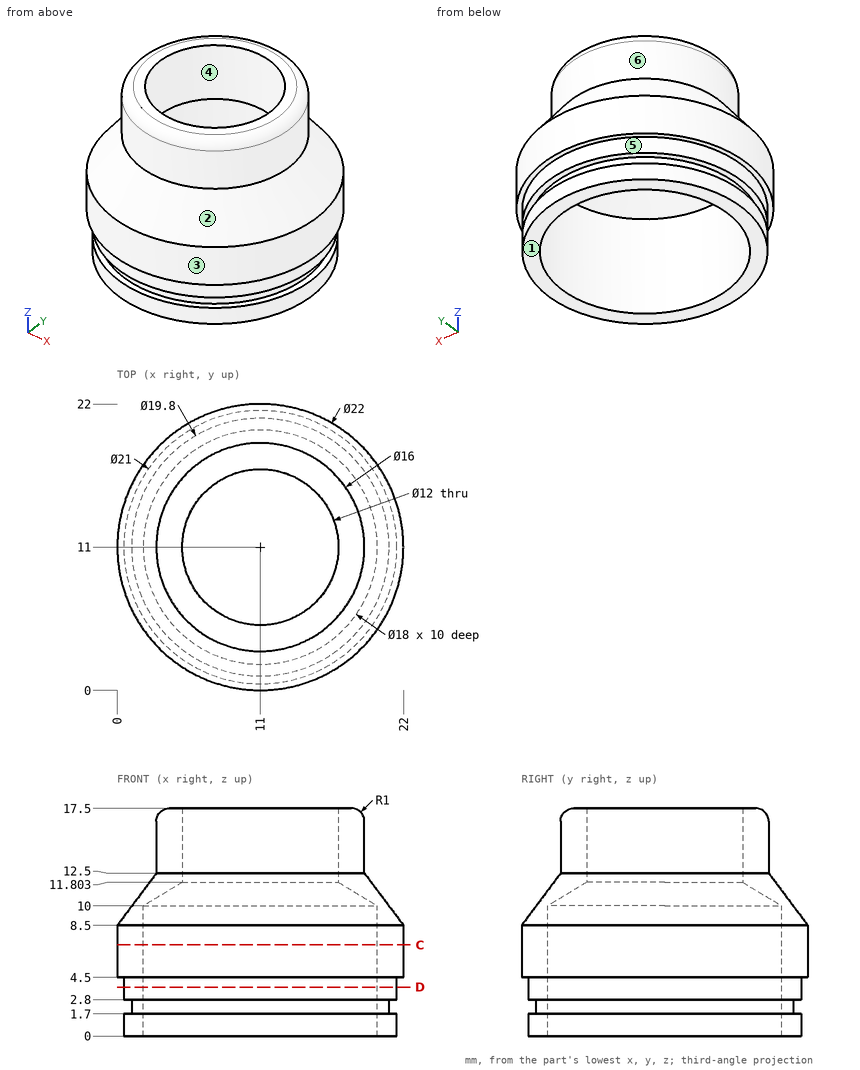
Input: dimensioned drawing with shaded views. Units: mm. Origin: part minimum x, y, z. A direction names the side the tool comes from. Round coordinates to 2 decimals unless told otherwise and drop trailing zeros. Loops run counter-clockwise (first coordinate to the right, second up) from the corner with the lowest first, then second, coordinate; pieces in that order, holes last.
1) Pull-direction query (Z, two-part tool) for the marked faces 1, 2 and 3; classes: released by +Z, released by -Z, zero draft, split by the parting line, or undercut.
Ans:
face 1: released by -Z
face 2: released by +Z
face 3: zero draft
2) Set-up query: the marked faces 4, 5 and 6. Return all of +Z, -Z, +X, -X, +Y, -Y with unobstructed straight access to the full face (end or side cutting, diameter ignored); none if empty.
Ans:
face 4: +Z, -Z
face 5: -Z
face 6: +Z
3) Section query D-D on z = 3.75. Return the cut outline in (x, y).
Ans:
outline: circle Ø21 at (11, 11); hole circle Ø18 at (11, 11)
4) Section query C-C on z = 7. Return the cut outline in (x, y).
Ans:
outline: circle Ø22 at (11, 11); hole circle Ø18 at (11, 11)
5) Pin query (flat end, axial travel): pin 1 (6.5 mm diameter, centred on x = 9, y = 13, fed in from -Z) (1 decimal); pin 2 (5 mm diameter, centred on y = 10, z = 15.5, fed in from -X); pin 3 (8 mm diameter, centred on y = 16.5, z = 3.5, fed in from +X). Return the tip coordinate at first contact, or that it passes through.
Ans:
pin 1: stops at z = 11.8
pin 2: stops at x = 3
pin 3: stops at x = 21.88
6) Material intervals for line 1 (Y direction, x = 11, z = 14.2); line 2 (Y direction, x = 11, z = 3.25); line 3 (X direction, y = 5.5, z = 14.25) (1 decimal), sorted ascending.
Ans:
line 1: y = 3 to 5, 17 to 19
line 2: y = 0.5 to 2, 20 to 21.5
line 3: x = 5.2 to 8.6, 13.4 to 16.8
